Build history of the part. All positions in model axes, mm. A direction names the side the tool comes from. Round coordinates to 2 decimals unless told otherwise and drop trailing zeros. Write each loop counter-clockwise with the first axis right and the second up, starting at its lowest first coordinate (ties: lowest second). Pieces come first, ordered by that corner, then holes.
Item 1: Band-saw the part on B-B, the plane z = 0. Write the cut outline in (x, y), then the cut area to 3 significant figures.
Item 2: Band-saw the part on C-C, the plane y = 4. Write the cut outline in (x, z).
Item 3: Band-saw the part on A-A, the plane x = 0. Write the cut outline in (y, z), then the cut area to 3 significant figures.
Item 4: 3-axis set-ups, long thin cutter, end or side, ignore diameter. For faces 4 (the flat face through (5, 1, -10)), 5 (the flat face through (3, 32, 3)): which of +Z, -Z, +X, -X, +Y, -Y reach the whole face in a straight line?
Item 5: Band-saw the part on D-D, the plane y = 22.5. Write the cut outline in (x, z), then the cut area to 3 significant figures.
Item 6: Mould opens along X. For faces 1 (the flat face through (2.5, 0, 2.8)), 2 (the cylindrical face through (3.233, 15.776, 1.341)), 3 (the cylindrical face through (-11.99, 0.49, 0.53)) say: +X half, -X half, draft (parallel to the pull), parting line (faces both ways), or undercut.
Item 7: Wall check: probe 1 along Z at (x, y) = (0, 23.5); probe 2 along Y at (x, z) = (-10.5, 4.5). Give the ranges that are in metal, low to high.
Item 8: Drop flat-ended pins along their axis: pin 1 Ø1 at (x, y) = (0.5, 28.5) entering from +Z; pin 2 Ø6 at (y, z) = (22, -6.5) entering from +X; pin 3 Ø5 at (x, z) = (2.5, -9) entering from -Y; pin 4 Ø5 at (x, y) = (6, 12) entering from +Z. Give the stop position or say it passes through.
```python
from build123d import *

# Parameters (mm, degrees)
CROQUIS1_R              = 7
CROQUIS1_R_2            = 3.5
SALIENTE_EXTRUIR1_DEPTH = 32
CROQUIS2_R              = 12
CROQUIS2_R_2            = 7
SALIENTE_EXTRUIR2_DEPTH = 1
REDONDEO1_R             = 4


with BuildPart() as part:
    # Croquis1 → Saliente-Extruir1 (new body)
    with BuildSketch(Plane(origin=(0, 0, 0), x_dir=(1, 0, 0), z_dir=(0, 1, 0))):
        Circle(CROQUIS1_R)
        Circle(CROQUIS1_R_2, mode=Mode.SUBTRACT)
    extrude(amount=SALIENTE_EXTRUIR1_DEPTH)

    # Croquis2 → Saliente-Extruir2 (add)
    with BuildSketch(Plane.XZ):
        Circle(CROQUIS2_R)
        Circle(CROQUIS2_R_2, mode=Mode.SUBTRACT)
    extrude(amount=-SALIENTE_EXTRUIR2_DEPTH)

    # Redondeo1
    redondeo1_edges = [part.edges().sort_by_distance(p)[0] for p in [
        (-7, 1, 0),
    ]]
    fillet(redondeo1_edges, radius=REDONDEO1_R)


solid = part.part
```
Results:
1. outline: (-12, 0) - (-3.5, 0) - (-3.5, 32) - (-7, 32) - (-7, 5) arc R4 cw to (-11, 1) - (-12, 1) - close; (3.5, 0) - (12, 0) - (12, 1) - (11, 1) arc R4 cw to (7, 5) - (7, 32) - (3.5, 32) - close
1. area: 241 mm2
2. outline: circle Ø14.25 at (0, 0); hole circle Ø7 at (0, 0)
3. outline: (0, -12) - (1, -12) - (1, -11) arc R4 cw to (5, -7) - (32, -7) - (32, -3.5) - (0, -3.5) - close; (0, 3.5) - (32, 3.5) - (32, 7) - (5, 7) arc R4 cw to (1, 11) - (1, 12) - (0, 12) - close
3. area: 241 mm2
4. face 4: +Y
4. face 5: +Z, -Z, +X, -X, +Y
5. outline: circle Ø14 at (0, 0); hole circle Ø7 at (0, 0)
5. area: 115 mm2
6. face 1: draft
6. face 2: undercut
6. face 3: parting line
7. probe 1: z = -7 to -3.5, 3.5 to 7
7. probe 2: y = 0 to 1
8. pin 1: stops at z = 7
8. pin 2: stops at x = 6.06
8. pin 3: stops at y = 0
8. pin 4: stops at z = 6.06
